Geometry check sheet. Reference: drawing and pictorial views, mm from the part's lowest x, y, z. Round coordinates to 2 decimals unless told otherwise and drop trailing zeros. Write each loop counter-clockwise with the first axis right and the second up, starting at its lowest first coordinate (ties: lowest second). Pieces come first, ordered by that corner, then holes. Notation, with made-up numbers: (21.25, -23.5) -> (28.25, -23.5) arc R28 cw to (28.25, 0.5) -> close; hole circle Ø7 at (-38, 51.5). An arc over 180 degrees is marked (long way). Write item = value, one per line.
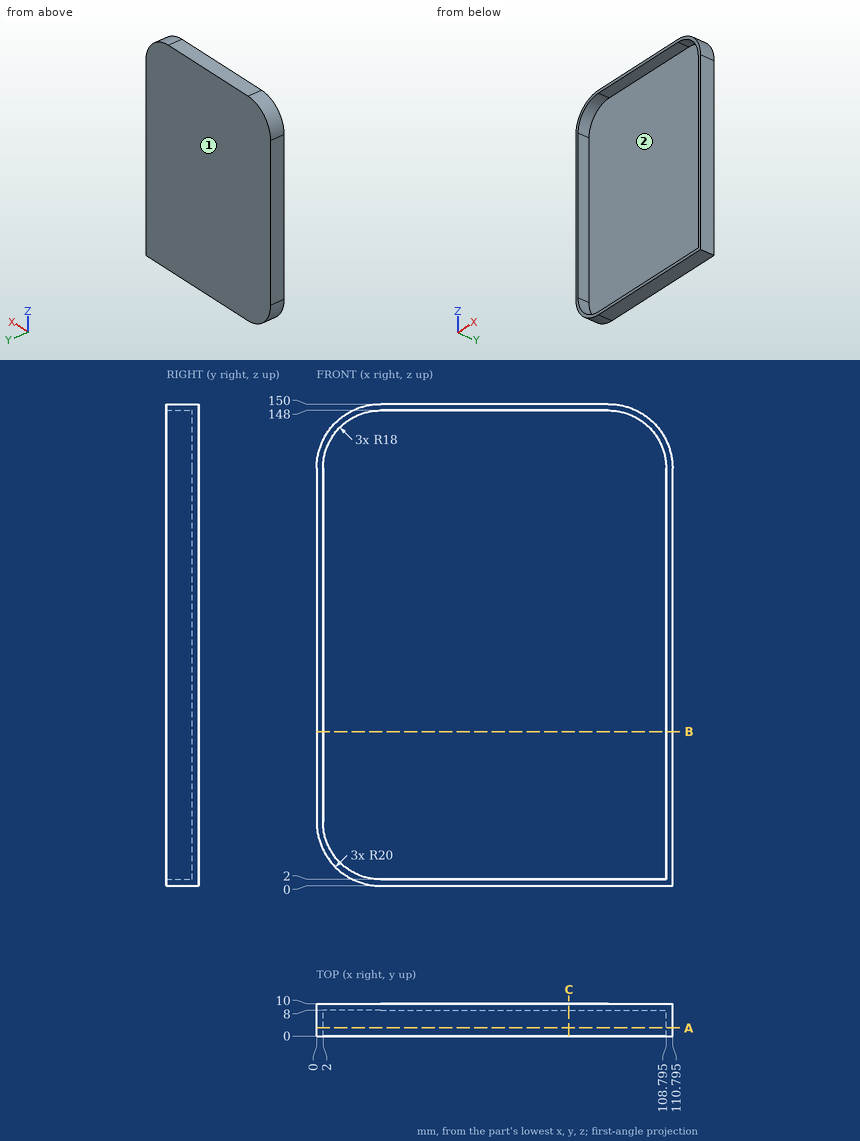
(1) Sectioned sample at B-B on z = 48. Enter the section's corners in (x, y) (1 decimal).
Worked answers:
outline = (0, 0) -> (2, 0) -> (2, 8) -> (108.8, 8) -> (108.8, 0) -> (110.8, 0) -> (110.8, 10) -> (0, 10) -> close
(2) Go/stop test with a flat-tipped pin: P1, Ø2, axis at x = 17.5, z = 104, coming from the -Y side. Record where the tip stops, or that it passes through.
Worked answers:
P1 = 8
(3) Sectioned sample at A-A on y = 2.5. Enter the section's corners in (x, z) (1 decimal).
Worked answers:
outline = (0, 20) arc R20 ccw to (20, 0) -> (110.8, 0) -> (110.8, 130) arc R20 ccw to (90.8, 150) -> (20, 150) arc R20 ccw to (0, 130) -> close; hole (2, 20) arc R18 ccw to (20, 2) -> (108.8, 2) -> (108.8, 130) arc R18 ccw to (90.8, 148) -> (20, 148) arc R18 ccw to (2, 130) -> close
(4) Sectioned sample at C-C on x = 78.5. Enter the section's corners in (y, z), then the cut area to 3 significant figures.
Worked answers:
outline = (0, 0) -> (10, 0) -> (10, 150) -> (0, 150) -> (0, 148) -> (8, 148) -> (8, 2) -> (0, 2) -> close
area = 332 mm²
(5) Release check for a two-part mould opening along Z. For the marked faces 1 and 2 record: pulls with the +Z half, pulls with the -Z half, needs draft (parallel to the pull), parting line crosses it, or undercut.
Worked answers:
face_1 = needs draft
face_2 = undercut
(6) Material ranges on L1, parallel to X at y = 3.5, z = 50.5 (1 decimal); L2, parallel to Z at x = 56.5, y = 1.75; L3, parallel to Y at x = 92.5, z = 12, recorded low to high. Write a range as [from, to].
Worked answers:
L1 = [0, 2], [108.8, 110.8]
L2 = [0, 2], [148, 150]
L3 = [8, 10]
